For this review, take the finished solid that the model builds, in its own axes (mm). A direction names the side the tool comes from. Give positions to 0.01 mm unless a question says otherwise; leave off trailing zeros. Order: outer loops, then holes, each group sorted by start corner. A loop starts at its lowest first (then second) coordinate and runs counter-clockwise, first axis right, second up.
Item 1: Machinability: for faces 4 (the flat face through (-29, 10, 46)), 5 (the flat face through (-13, 11, 4)), 6 (the flat face through (20, 7.5, 8)), 7 (the flat face through (-2, 13, 13)), which of the approach directions +Z, -Z, +X, -X, +Y, -Y give a long, thin tool a straight path to every point of the face, cutting with its end or side? Answer none if there is none.
Item 2: Consider section B-B (z = 46). Give the boundary of the cut face in (x, y).
Item 3: The part is to be moulded in two halves that separate along Z. For faces 1 (the flat face through (-13, 11, 36)), 2 (the flat face through (-17.8, 23.49, 39.15)), 3 (the flat face through (-12, 15, 11)), say which applies: released by +Z, released by -Z, zero draft, split by the parting line, or undercut.
Item 4: Consider section D-D (x = 31). Give the boundary of the cut face in (y, z).
Item 5: Consider section C-C (z = 4). Give the boundary of the cut face in (x, y).
Item 6: For P1, Ø5.5, axis at x = -30, z = 47.5, coming from the +Y side; P2, Ø2, axis at x = -2.75, z = 46, coming from the -Y side; P3, Ø2.5, axis at x = 11.5, y = -10.5, coming from the +Z side, all flat-tipped, find the tip position at first contact; note any pin that passes through.
Item 7: Consider section A-A (x = -2.75). Give the boundary of the cut face in (y, z).
Item 8: For probe 1 along Y at (x, z) = (-26, 20); probe 2 along X at (y, z) = (12, 46); probe 3 along Z at (x, y) = (-30.25, 11.55), list the stretches that pass through material, from the lowest coordinate up.
```python
from build123d import *

# Parameters (mm, degrees)
PAD_DEPTH       = 15
SKETCH001_W     = 40
SKETCH001_H     = 15
PAD001_DEPTH    = 10
SKETCH002_R     = 2
POCKET_DEPTH    = 20
SKETCH003_W     = 5
SKETCH003_H     = 5
PAD002_DEPTH    = 12
SKETCH004_R     = 0.9
POCKET001_DEPTH = 5.001
PAD003_DEPTH    = 33
POCKET002_DEPTH = 73.001
CHAMFER_SIZE    = 2
CHAMFER001_SIZE = 2
CHAMFER002_SIZE = 1
CHAMFER003_SIZE = 4
SKETCH007_R     = 3.5
POCKET003_DEPTH = 8
SKETCH008_R     = 3
POCKET004_DEPTH = 14
CHAMFER004_SIZE = 3


with BuildPart() as part:
    # Sketch → Pad (new body, symmetric)
    with BuildSketch(Plane.XZ):
        Polygon((-33, 40), (-33, 0), (40, 0), (40, 3), (0, 3), (0, 40), align=None)
    extrude(amount=PAD_DEPTH, both=True)

    # Sketch001 (on Face4 of Pad) → Pad001 (join)
    with BuildSketch(Plane(origin=(0, 0, 3), x_dir=(-1, 0, 0), z_dir=(0, 0, 1))):
        with Locations((-20, 0)):
            Rectangle(SKETCH001_W, SKETCH001_H)
    extrude(amount=PAD001_DEPTH)

    # Sketch002 (on Face1 of Pad001) → Pocket (cut)
    with BuildSketch(Plane(origin=(-33, 0, 0), x_dir=(0, 0, -1), z_dir=(-1, 0, 0))):
        with Locations((-36, 11.0000000011)):
            Circle(SKETCH002_R)
        with Locations((-20, 11.0000000011)):
            Circle(SKETCH002_R)
        with Locations((-4, 11)):
            Circle(SKETCH002_R)
        with Locations((-4, -11)):
            Circle(SKETCH002_R)
        with Locations((-20, -11.0000000011)):
            Circle(SKETCH002_R)
        with Locations((-36, -11.0000000011)):
            Circle(SKETCH002_R)
    extrude(amount=-POCKET_DEPTH, mode=Mode.SUBTRACT)

    # Sketch003 (on Face2 of Pocket) → Pad002 (join)
    with BuildSketch(Plane(origin=(0, 0, 40), x_dir=(-1, 0, 0), z_dir=(0, 0, 1))):
        with Locations((2.5, -12.5)):
            Rectangle(SKETCH003_W, SKETCH003_H)
        with Locations((30.5, -12.5)):
            Rectangle(SKETCH003_W, SKETCH003_H)
    extrude(amount=PAD002_DEPTH)

    # Sketch004 (on Face6 of Pad002) → Pocket001 (cut, through all)
    with BuildSketch(Plane.XZ.offset(-10)):
        with Locations((-30.25, 46)):
            Circle(SKETCH004_R)
        with Locations((-2.75, 46)):
            Circle(SKETCH004_R)
    extrude(amount=-POCKET001_DEPTH, mode=Mode.SUBTRACT)

    # Sketch005 (on Face9 of Pocket001) → Pad003 (join)
    with BuildSketch(Plane(origin=(0, 0, 0), x_dir=(0, 0, 1), z_dir=(1, 0, 0))):
        Polygon((22.6794919243, -15), (40, -25), (40, -15), align=None)
    extrude(amount=-PAD003_DEPTH)

    # Sketch006 (on Face22 of Pad003) → Pocket002 (cut, through all)
    with BuildSketch(Plane(origin=(-33, 0, 0), x_dir=(0, 0, -1), z_dir=(-1, 0, 0))):
        Polygon((-40, 5), (-22.6794919243, 15), (-40, 15), align=None)
    extrude(amount=-POCKET002_DEPTH, mode=Mode.SUBTRACT)

    # Chamfer
    chamfer_edges = [part.edges().sort_by_distance(p)[0] for p in [
        (-16.5, 25, 40),
    ]]
    chamfer(chamfer_edges, length=CHAMFER_SIZE)

    # Chamfer001
    chamfer001_edges = [part.edges().sort_by_distance(p)[0] for p in [
        (40, -15, 1.5),
        (40, 15, 1.5),
    ]]
    chamfer(chamfer001_edges, length=CHAMFER001_SIZE)

    # Chamfer002
    chamfer002_edges = [part.edges().sort_by_distance(p)[0] for p in [
        (-33, -15, 11.339746),
        (-33, -10, 31.339746),
        (-33, 15, 11.339746),
        (-33, 19.5, 30.473721),
        (-33, 23.5, 39.133975),
    ]]
    chamfer(chamfer002_edges, length=CHAMFER002_SIZE)

    # Chamfer003
    chamfer003_edges = [part.edges().sort_by_distance(p)[0] for p in [
        (0, -15, 12.839746),
        (0, -10, 31.339746),
        (0, 19.5, 30.473721),
        (0, 15, 12.839746),
        (0, 23.5, 39.133975),
    ]]
    chamfer(chamfer003_edges, length=CHAMFER003_SIZE)

    # Sketch007 (on Face38 of Chamfer003) → Pocket003 (cut)
    with BuildSketch(Plane(origin=(0, -21.0705080757, 12.1650635095), x_dir=(1, 0, 0), z_dir=(0, -0.8660254038, 0.5))):
        with Locations((-10, 22.1410161514)):
            Circle(SKETCH007_R)
    extrude(amount=-POCKET003_DEPTH, mode=Mode.SUBTRACT)

    # Sketch008 (on Face11 of Pocket003) → Pocket004 (cut)
    with BuildSketch(Plane(origin=(0, 0, 0), x_dir=(0, 0, 1), z_dir=(1, 0, 0))):
        with Locations((27.330492, 2.925061)):
            Circle(SKETCH008_R)
    extrude(amount=-POCKET004_DEPTH, mode=Mode.SUBTRACT)

    # Chamfer004
    chamfer004_edges = [part.edges().sort_by_distance(p)[0] for p in [
        (-2.5, 15, 40),
        (-30.5, 15, 40),
    ]]
    chamfer(chamfer004_edges, length=CHAMFER004_SIZE)


solid = part.part
```
Resolved:
1. face 4: +Z, +X, -X, -Y
1. face 5: -X
1. face 6: +Z, +X, +Y
1. face 7: +X, +Y
2. outline: (-33, 10) - (-31.15, 10) - (-31.15, 15) - (-33, 15) - close; (-29.35, 10) - (-28, 10) - (-28, 15) - (-29.35, 15) - close; (-5, 10) - (-3.65, 10) - (-3.65, 15) - (-5, 15) - close; (-1.85, 10) - (0, 10) - (0, 15) - (-1.85, 15) - close
3. face 1: undercut
3. face 2: released by +Z
3. face 3: zero draft
4. outline: (-15, 0) - (15, 0) - (15, 3) - (7.5, 3) - (7.5, 13) - (-7.5, 13) - (-7.5, 3) - (-15, 3) - close
5. outline: (-33, -14) - (-32, -15) - (-4, -15) - (0, -11) - (0, -7.5) - (40, -7.5) - (40, 7.5) - (0, 7.5) - (0, 11) - (-4, 15) - (-32, 15) - (-33, 14) - (-33, 13) - (-13, 13) - (-13, 9) - (-33, 9) - (-33, -9) - (-13, -9) - (-13, -13) - (-33, -13) - close
6. P1: stops at y = 15
6. P2: stops at y = 10
6. P3: stops at z = 3
7. outline: (-15, 0) - (15, 0) - (15, 3) - (13.75, 3) - (13.75, 23.01) - (22.56, 38.27) - (21.56, 40) - (18, 40) - (15, 43) - (15, 45.1) - (10, 45.1) - (10, 40) - (-3.56, 40) - (-13.75, 22.34) - (-13.75, 3) - (-15, 3) - close; (10, 46.9) - (15, 46.9) - (15, 52) - (10, 52) - close; hole circle Ø6 at (-2.93, 27.33)
8. probe 1: y = -15 to -13, -9 to 9, 13 to 15
8. probe 2: x = -33 to -31.15, -29.35 to -28, -5 to -3.65, -1.85 to 0
8. probe 3: z = 0 to 2.08, 5.92 to 18.08, 21.92 to 34.08, 37.92 to 45.1, 46.9 to 52
